Verification items for the finished model (mm, model axes). Round coordinates to 2 decimals unless told otherwise and drop trailing zeros. Write item = value, one per line.
```python
from build123d import *
from build123d.topology import SkipClean

# Parameters (mm, degrees)
SKETCH2_R           = 175
SKETCH2_R_2         = 5
BOSS_EXTRUDE1_DEPTH = 15
CHAMFER1_SIZE       = 5
FILLET1_R           = 5
FILLET2_R           = 5
BOSS_EXTRUDE2_START = 22
BOSS_EXTRUDE2_DEPTH = 22


with BuildPart() as part:
    # Sketch2 → Boss-Extrude1 (new, symmetric)
    with BuildSketch(Plane.XY):
        Circle(SKETCH2_R)
        Polygon((16.339745962, -48.301270189), (33.660254038, -38.301270189), (79.557938048, -93), (32.608753123, -93), align=None, mode=Mode.SUBTRACT)
        Polygon((10, -50), (17.58206017, -93), (-17.58206017, -93), (-10, -50), align=None, mode=Mode.SUBTRACT)
        Polygon((-16.339745962, -48.301270189), (-32.608753123, -93), (-79.557938048, -93), (-33.660254038, -38.301270189), align=None, mode=Mode.SUBTRACT)
        with BuildLine():
            Line((-50, 10), (-50, -10))
            Line((-50, -10), (-137.66589003, -25.4578617))
            ThreePointArc((-137.66589003, -25.4578617), (-140, 0), (-137.66589003, 25.4578617))
            Line((-137.66589003, 25.4578617), (-50, 10))
        make_face(mode=Mode.SUBTRACT)
        with BuildLine():
            Line((-48.301270189, -16.339745962), (-38.301270189, -33.660254038))
            Line((-38.301270189, -33.660254038), (-106.49322715, -90.880099973))
            ThreePointArc((-106.49322715, -90.880099973), (-121.24355653, -70), (-131.95108885, -46.785790057))
            Line((-131.95108885, -46.785790057), (-48.301270189, -16.339745962))
        make_face(mode=Mode.SUBTRACT)
        with BuildLine():
            Line((38.301270189, -33.660254038), (48.301270189, -16.339745962))
            Line((48.301270189, -16.339745962), (131.95108885, -46.785790057))
            ThreePointArc((131.95108885, -46.785790057), (121.24355653, -70), (106.49322715, -90.880099973))
            Line((106.49322715, -90.880099973), (38.301270189, -33.660254038))
        make_face(mode=Mode.SUBTRACT)
        with Locations((32.7390252, -8.772395363)):
            Circle(SKETCH2_R_2, mode=Mode.SUBTRACT)
        with BuildLine():
            Line((-38.301270189, 33.660254038), (-48.301270189, 16.339745962))
            Line((-48.301270189, 16.339745962), (-131.95108885, 46.785790057))
            ThreePointArc((-131.95108885, 46.785790057), (-121.24355653, 70), (-106.49322715, 90.880099973))
            Line((-106.49322715, 90.880099973), (-38.301270189, 33.660254038))
        make_face(mode=Mode.SUBTRACT)
        with BuildLine():
            Line((-16.339745962, 48.301270189), (-33.660254038, 38.301270189))
            Line((-33.660254038, 38.301270189), (-90.880099973, 106.49322715))
            ThreePointArc((-90.880099973, 106.49322715), (-70, 121.24355653), (-46.785790057, 131.95108885))
            Line((-46.785790057, 131.95108885), (-16.339745962, 48.301270189))
        make_face(mode=Mode.SUBTRACT)
        with BuildLine():
            Line((10, 50), (-10, 50))
            Line((-10, 50), (-25.4578617, 137.66589003))
            ThreePointArc((-25.4578617, 137.66589003), (0, 140), (25.4578617, 137.66589003))
            Line((25.4578617, 137.66589003), (10, 50))
        make_face(mode=Mode.SUBTRACT)
        with BuildLine():
            ThreePointArc((2.5, 12.247448714), (0, -12.5), (-2.5, 12.247448714))
            Line((-2.5, 12.247448714), (-2.5, 7.247448714))
            Line((-2.5, 7.247448714), (2.5, 7.247448714))
            Line((2.5, 7.247448714), (2.5, 12.247448714))
        make_face(mode=Mode.SUBTRACT)
        with BuildLine():
            Line((48.301270189, 16.339745962), (38.301270189, 33.660254038))
            Line((38.301270189, 33.660254038), (106.49322715, 90.880099973))
            ThreePointArc((106.49322715, 90.880099973), (121.24355653, 70), (131.95108885, 46.785790057))
            Line((131.95108885, 46.785790057), (48.301270189, 16.339745962))
        make_face(mode=Mode.SUBTRACT)
        with BuildLine():
            Line((33.660254038, 38.301270189), (16.339745962, 48.301270189))
            Line((16.339745962, 48.301270189), (46.785790057, 131.95108885))
            ThreePointArc((46.785790057, 131.95108885), (70, 121.24355653), (90.880099973, 106.49322715))
            Line((90.880099973, 106.49322715), (33.660254038, 38.301270189))
        make_face(mode=Mode.SUBTRACT)
        with BuildLine():
            Line((50, -10), (50, 10))
            Line((50, 10), (137.66589003, 25.4578617))
            ThreePointArc((137.66589003, 25.4578617), (140, 0), (137.66589003, -25.4578617))
            Line((137.66589003, -25.4578617), (50, -10))
        make_face(mode=Mode.SUBTRACT)
    extrude(amount=BOSS_EXTRUDE1_DEPTH, both=True)

    # Chamfer1
    chamfer1_edges = [part.edges().sort_by_distance(p)[0] for p in [
        (-175, 0, 15),
        (-175, 0, -15),
    ]]
    chamfer(chamfer1_edges, length=CHAMFER1_SIZE)

    # Fillet1
    fillet1_edges = [part.edges().sort_by_distance(p)[0] for p in [
        (-50, -10, 0),
        (-50, 10, 0),
        (-38.301270189, -33.660254038, 0),
        (-48.301270189, -16.339745962, 0),
        (48.301270189, -16.339745962, 0),
        (38.301270189, -33.660254038, 0),
        (50, 10, 0),
        (50, -10, 0),
        (38.301270189, 33.660254038, 0),
        (48.301270189, 16.339745962, 0),
        (16.339745962, 48.301270189, 0),
        (33.660254038, 38.301270189, 0),
        (-10, 50, 0),
        (10, 50, 0),
        (33.660254038, -38.301270189, 0),
        (16.339745962, -48.301270189, 0),
        (10, -50, 0),
        (-10, -50, 0),
        (-16.339745962, -48.301270189, 0),
        (-33.660254038, -38.301270189, 0),
        (-33.660254038, 38.301270189, 0),
        (-16.339745962, 48.301270189, 0),
        (-48.301270189, 16.339745962, 0),
        (-38.301270189, 33.660254038, 0),
    ]]
    fillet(fillet1_edges, radius=FILLET1_R)

    # Fillet2
    fillet2_edges = [part.edges().sort_by_distance(p)[0] for p in [
        (-137.66589003, 25.4578617, 0),
        (-137.66589003, -25.4578617, 0),
        (-131.95108885, -46.785790057, 0),
        (-106.49322715, -90.880099973, 0),
        (106.49322715, -90.880099973, 0),
        (131.95108885, -46.785790057, 0),
        (137.66589003, -25.4578617, 0),
        (137.66589003, 25.4578617, 0),
        (131.95108885, 46.785790057, 0),
        (106.49322715, 90.880099973, 0),
        (90.880099973, 106.49322715, 0),
        (46.785790057, 131.95108885, 0),
        (25.4578617, 137.66589003, 0),
        (-25.4578617, 137.66589003, 0),
        (32.608753123, -93, 0),
        (79.557938048, -93, 0),
        (-17.58206017, -93, 0),
        (17.58206017, -93, 0),
        (-79.557938048, -93, 0),
        (-32.608753123, -93, 0),
        (-46.785790057, 131.95108885, 0),
        (-90.880099973, 106.49322715, 0),
        (-106.49322715, 90.880099973, 0),
        (-131.95108885, 46.785790057, 0),
    ]]
    fillet(fillet2_edges, radius=FILLET2_R)

    # Sketch2_3 → Boss-Extrude2 (add)
    with SkipClean():  # the faces are left unmerged after this step: merging them gives an invalid solid
        with BuildSketch(Plane.XY.offset(BOSS_EXTRUDE2_START)):
            with BuildLine():
                Line((148.243043682, -93), (79.557938048, -93))
                Line((79.557938048, -93), (90.880099973, -106.49322715))
                ThreePointArc((90.880099973, -106.49322715), (70, -121.24355653), (46.785790057, -131.95108885))
                Line((46.785790057, -131.95108885), (32.608753123, -93))
                Line((32.608753123, -93), (17.58206017, -93))
                Line((17.58206017, -93), (25.4578617, -137.66589003))
                ThreePointArc((25.4578617, -137.66589003), (0, -140), (-25.4578617, -137.66589003))
                Line((-25.4578617, -137.66589003), (-17.58206017, -93))
                Line((-17.58206017, -93), (-32.608753123, -93))
                Line((-32.608753123, -93), (-46.785790057, -131.95108885))
                ThreePointArc((-46.785790057, -131.95108885), (-70, -121.24355653), (-90.880099973, -106.49322715))
                Line((-90.880099973, -106.49322715), (-79.557938048, -93))
                Line((-79.557938048, -93), (-148.243043682, -93))
                ThreePointArc((-148.243043682, -93), (0, -175), (148.243043682, -93))
            make_face()
            with BuildLine():
                Line((-32.608753123, -93), (-79.557938048, -93))
                Line((-79.557938048, -93), (-90.880099973, -106.49322715))
                ThreePointArc((-90.880099973, -106.49322715), (-70, -121.24355653), (-46.785790057, -131.95108885))
                Line((-46.785790057, -131.95108885), (-32.608753123, -93))
            make_face()
            with BuildLine():
                Line((25.4578617, -137.66589003), (17.58206017, -93))
                Line((17.58206017, -93), (-17.58206017, -93))
                Line((-17.58206017, -93), (-25.4578617, -137.66589003))
                ThreePointArc((-25.4578617, -137.66589003), (0, -140), (25.4578617, -137.66589003))
            make_face()
            with BuildLine():
                Line((90.880099973, -106.49322715), (79.557938048, -93))
                Line((79.557938048, -93), (32.608753123, -93))
                Line((32.608753123, -93), (46.785790057, -131.95108885))
                ThreePointArc((46.785790057, -131.95108885), (70, -121.24355653), (90.880099973, -106.49322715))
            make_face()
        extrude(amount=-BOSS_EXTRUDE2_DEPTH)


solid = part.part
```
(1) Draft check along Y on faces 1 (the face through (24.93, -43.34, 0.21)), 2 (the face through (-121.1, -70.25, 0.21)). Enter one of: released by +Y, released by -Y, zero draft, split by the parting line, or undercut.
Filled sheet:
face_1 = undercut
face_2 = undercut
(2) Material ranges on probe 1 along X at (y, z) = (125, 8.5); probe 2 along Y at (x, z) = (112.5, -4.5); probe 3 along Y at (x, z) = (-57.5, -12), recorded low to high. Write a range as from..to.
Filled sheet:
probe_1 = -122.47..-63.05, -44.26..-23.22, 23.22..44.26, 63.05..122.47
probe_2 = -134.05..-83.33, -39.71..-21.02, 21.02..39.71, 83.33..134.05
probe_3 = -163.16..-93, -66.71..-49.77, -19.69..-11.32, 11.32..19.69, 49.77..66.71, 127.65..163.16
(3) Go/stop test with flat-tipped pins: pin 1 Ø7.5 at (x, z) = (48, 18) entering from +Y; pin 2 Ø9.5 at (x, z) = (-105, 13) entering from +Y; pin 3 Ø1 at (x, z) = (-76, -5) entering from -Y. Record where each tip stops, or that it passes through.
Filled sheet:
pin_1 = 164.01
pin_2 = 142.69
pin_3 = -157.88
(4) Sectioned sample at A-A, the plane z = 4. Count the separate pieces of the cut face and the enclosed holes in it, and give its area (3 significant figures).
Filled sheet:
separate_pieces = 1
enclosed_holes = 14
area = 62,500 mm2
